Here's how the part is built. I have some questions about the finished solid (model axes, mm). A direction names the side the tool comes from. Round coordinates to 2 decimals unless told otherwise and drop trailing zeros. Order: outer loops, then holes, each group sorted by start corner. A loop starts at its lowest first (then second) coordinate and runs counter-clockwise, first axis right, second up.
```python
from build123d import *

# Parameters (mm, degrees)
SKETCH_1_W                = 24.86
SKETCH_1_H                = 41.68
SKETCH_1_R                = 0.75
EXTRUDE_2_DEPTH           = 2
SKETCH_4_W                = 2.869231424
SKETCH_4_H                = 4.001531821
SKETCH_4_W_2              = 2.43
SKETCH_4_H_2              = 4
EXTRUDE_3_DEPTH           = 24
SKETCH_8_W                = 3.310255182
SKETCH_8_H                = 4.675588029
SKETCH_8_W_2              = 3.47
EXTRUDE_5_DEPTH           = 16.03
FILLET_5_R                = 2.4
FILLET_6_R                = 2.4
FILLET_7_R                = 2.4
FILLET_8_R                = 2.4
CUT_EXTRUDE_7_DEPTH       = 16.03
CUT_EXTRUDE_7_DEPTH_BACK  = 16.03
SKETCH_13_R               = 1.236878532
CUT_EXTRUDE_8_DEPTH       = 16.03
CUT_EXTRUDE_8_DEPTH_BACK  = 16.03
SKETCH_5_R                = 1.45
CUT_EXTRUDE_9_DEPTH       = 16.03
CUT_EXTRUDE_9_DEPTH_BACK  = 16.03
SKETCH_14_R               = 1.4
SKETCH_16_W               = 16.135324728
SKETCH_16_H               = 3.096678483
EXTRUDE_8_DEPTH           = 10
FILLET_10_R               = 5
FILLET_13_R               = 5
SKETCH_17_W               = 2.433704545
SKETCH_17_H               = 5.946026496
SKETCH_17_W_2             = 1.564461462
SKETCH_17_H_2             = 6
EXTRUDE_9_DEPTH           = 15
CHAMFER_1_SIZE            = 10
CHAMFER_2_SIZE            = 10
CUT_EXTRUDE_16_DEPTH      = 10
CUT_EXTRUDE_16_DEPTH_BACK = 10
SKETCH_19_W               = 2.68
SKETCH_19_H               = 23.433804394
CUT_EXTRUDE_17_DEPTH      = 10
CUT_EXTRUDE_17_DEPTH_BACK = 10
SKETCH_18_W               = 2.24898196
SKETCH_18_H               = 30.410340658
FILLET_17_R               = 2
FILLET_18_R               = 2
FILLET_19_R               = 1


with BuildPart() as part:
    # 草图1 → 凸台-拉伸2 (new body)
    with BuildSketch(Plane(origin=(0, 0, 0), x_dir=(1, 0, 0), z_dir=(0, 1, 0))):
        Rectangle(SKETCH_1_W, SKETCH_1_H)
        with Locations(Location((-10.842762007, 19.642978565, 0), (0, 0, 270))):
            Circle(SKETCH_1_R, mode=Mode.SUBTRACT)
        with Locations(Location((10.87870886, 19.719816311, 0), (0, 0, 270))):
            Circle(SKETCH_1_R, mode=Mode.SUBTRACT)
        with Locations(Location((-10.713936696, -19.568538996, 0), (0, 0, 270))):
            Circle(SKETCH_1_R, mode=Mode.SUBTRACT)
        with Locations(Location((10.87870886, -19.568538996, 0), (0, 0, 270))):
            Circle(SKETCH_1_R, mode=Mode.SUBTRACT)
    extrude(amount=EXTRUDE_2_DEPTH)

    # 草图4 → 凸台-拉伸3 (add)
    with BuildSketch(Plane(origin=(0, 0, 0), x_dir=(1, 0, 0), z_dir=(0, 1, 0))):
        with Locations((-10.995384288, -16.41923409)):
            Rectangle(SKETCH_4_W, SKETCH_4_H)
        with Locations((11.215, -16.42)):
            Rectangle(SKETCH_4_W_2, SKETCH_4_H_2)
    extrude(amount=EXTRUDE_3_DEPTH)

    # 草图8 → 凸台-拉伸5 (add)
    with BuildSketch(Plane(origin=(0, 0, 0), x_dir=(1, 0, 0), z_dir=(0, 1, 0))):
        with Locations((-1.655127591, 18.102205985)):
            Rectangle(SKETCH_8_W, SKETCH_8_H)
        with Locations((4.770502505, 18.102205985)):
            Rectangle(SKETCH_8_W_2, SKETCH_8_H)
    extrude(amount=EXTRUDE_5_DEPTH)

    # 圆角5
    fillet_5_edges = [part.edges().sort_by_distance(p)[0] for p in [
        (-1.655127591, 16.03, -15.764411971),
    ]]
    fillet(fillet_5_edges, radius=FILLET_5_R)

    # 圆角6
    fillet_6_edges = [part.edges().sort_by_distance(p)[0] for p in [
        (4.770502505, 16.03, -15.764411971),
    ]]
    fillet(fillet_6_edges, radius=FILLET_6_R)

    # 圆角7
    # the kernel refuses this fillet: 2.4 mm, written as the material it takes off along each edge
    with BuildSketch(Plane(origin=(-2.956430437, 16.03, -20.44), x_dir=(0, 0, 1), z_dir=(1, 0, 0))) as fillet_7_piece_1_section:
        with BuildLine():
            CenterArc((2.4, 2.396773177), FILLET_7_R, 180, 87.028551133)
            Line((0, 2.396773177), (0, 0))
            Line((0, 0), (2.275588029, 0))
        make_face()
    fillet_7_piece_1 = extrude(amount=15.453865884, mode=Mode.PRIVATE)
    fillet_7_piece_1 = split(fillet_7_piece_1, bisect_by=Plane(origin=(0, 16.03, -20.44), z_dir=(1, 0, 0)), keep=Keep.TOP, mode=Mode.PRIVATE)
    add(fillet_7_piece_1, mode=Mode.SUBTRACT)

    # 圆角8
    # the kernel refuses this fillet: 2.4 mm, written as the material it takes off along each edge
    with BuildSketch(Plane(origin=(-9.302188124, 16.03, -20.44), x_dir=(0, 0, 1), z_dir=(1, 0, 0))) as fillet_8_piece_1:
        with BuildLine():
            CenterArc((2.4, 2.396773177), FILLET_8_R, 180, 87.028551133)
            Line((0, 2.396773177), (-0.048, 2.396773177))
            Line((-0.048, 2.396773177), (-0.048, 0))
            Line((-0.048, 0), (0, -0.048))
            ThreePointArc((0, -0.048), (1.137794014, -0.048), (2.273099789, -0.047935464))
            Line((2.273099789, -0.047935464), (2.275588029, 0))
        make_face()
    extrude(amount=15.294121066, mode=Mode.SUBTRACT)

    # 草图13 → 切除-拉伸7 (cut, two sides: drawn at the far end of the back side and taken through both)
    with BuildSketch(Plane(origin=(0, 0, 0), x_dir=(0, 0, -1), z_dir=(1, 0, 0)).offset(-CUT_EXTRUDE_7_DEPTH_BACK)):
        with Locations(Location((18.052862707, 13.197698645, 0), (0, 0, 180))):
            Circle(SKETCH_13_R)
    extrude(amount=CUT_EXTRUDE_7_DEPTH + CUT_EXTRUDE_7_DEPTH_BACK, mode=Mode.SUBTRACT)

    # 草图5 → 切除-拉伸8 (cut, two sides: drawn at the far end of the back side and taken through both)
    with BuildSketch(Plane(origin=(0, 0, 0), x_dir=(0, 0, -1), z_dir=(1, 0, 0)).offset(-CUT_EXTRUDE_8_DEPTH_BACK)):
        with Locations(Location((-16.419309005, 4.2, 0), (0, 0, 180))):
            Circle(SKETCH_5_R)
    extrude(amount=CUT_EXTRUDE_8_DEPTH + CUT_EXTRUDE_8_DEPTH_BACK, mode=Mode.SUBTRACT)

    # 草图14 → 切除-拉伸9 (cut, two sides: drawn at the far end of the back side and taken through both)
    with BuildSketch(Plane(origin=(0, 0, 0), x_dir=(0, 0, -1), z_dir=(1, 0, 0)).offset(-CUT_EXTRUDE_9_DEPTH_BACK)):
        with Locations(Location((-16.419309005, 22.241125132, 0), (0, 0, 180))):
            Circle(SKETCH_14_R)
    extrude(amount=CUT_EXTRUDE_9_DEPTH + CUT_EXTRUDE_9_DEPTH_BACK, mode=Mode.SUBTRACT)

    # 草图16 → 凸台-拉伸8 (add)
    with BuildSketch(Plane(origin=(0, 0, 0), x_dir=(1, 0, 0), z_dir=(0, 1, 0))):
        with Locations((1.276700778, 17.221878583)):
            Rectangle(SKETCH_16_W, SKETCH_16_H)
    extrude(amount=EXTRUDE_8_DEPTH)

    # 圆角10
    fillet_10_edges = [part.edges().sort_by_distance(p)[0] for p in [
        (-6.790961586, 10, -17.221878582),
    ]]
    fillet(fillet_10_edges, radius=FILLET_10_R)

    # 圆角13
    fillet_13_edges = [part.edges().sort_by_distance(p)[0] for p in [
        (9.344363142, 10, -17.221878582),
    ]]
    fillet(fillet_13_edges, radius=FILLET_13_R)

    # 草图17 → 凸台-拉伸9 (add)
    with BuildSketch(Plane(origin=(0, 0, 0), x_dir=(1, 0, 0), z_dir=(0, 1, 0))):
        with Locations((-11.213147728, -11.445454931)):
            Rectangle(SKETCH_17_W, SKETCH_17_H)
        with Locations((11.647769269, -11.42)):
            Rectangle(SKETCH_17_W_2, SKETCH_17_H_2)
    extrude(amount=EXTRUDE_9_DEPTH)

    # 倒角1
    # the kernel refuses this chamfer: 10 mm, written as the material it takes off along each edge
    with BuildSketch(Plane(origin=(-38.14682988, 15, 8.472441683), x_dir=(0, 0, 1), z_dir=(1, 0, 0))) as chamfer_1_piece_1_section:
        Polygon((CHAMFER_1_SIZE, 0), (0, CHAMFER_1_SIZE), (0, 0), align=None)
    chamfer_1_piece_1 = extrude(amount=53.867364305, mode=Mode.PRIVATE)
    chamfer_1_piece_1 = split(chamfer_1_piece_1, bisect_by=Plane(origin=(-38.14682988, 15, 14.418468179), z_dir=(0, 0, -1)), keep=Keep.TOP, mode=Mode.PRIVATE)
    chamfer_1_piece_1 = split(chamfer_1_piece_1, bisect_by=Plane(origin=(10, 15, 8.472441683), z_dir=(-1, 0, 0)), keep=Keep.TOP, mode=Mode.PRIVATE)
    add(chamfer_1_piece_1, mode=Mode.SUBTRACT)

    # 倒角2
    # the kernel refuses this chamfer: 10 mm, written as the material it takes off along each edge
    with BuildSketch(Plane(origin=(38.14682988, 15, 8.42), x_dir=(0, 0, 1), z_dir=(-1, 0, 0))) as chamfer_2_piece_1_section:
        Polygon((CHAMFER_2_SIZE, 0), (0, -CHAMFER_2_SIZE), (0, 0), align=None)
    chamfer_2_piece_1 = extrude(amount=52.998121222, mode=Mode.PRIVATE)
    chamfer_2_piece_1 = split(chamfer_2_piece_1, bisect_by=Plane(origin=(38.14682988, 15, 14.42), z_dir=(0, 0, -1)), keep=Keep.TOP, mode=Mode.PRIVATE)
    chamfer_2_piece_1 = split(chamfer_2_piece_1, bisect_by=Plane(origin=(10, 15, 8.42), z_dir=(1, 0, 0)), keep=Keep.TOP, mode=Mode.PRIVATE)
    add(chamfer_2_piece_1, mode=Mode.SUBTRACT)

    # 草图19 → 切除-拉伸16 (cut, two sides: drawn at the far end of the back side and taken through both)
    with BuildSketch(Plane(origin=(0, 0, 0), x_dir=(1, 0, 0), z_dir=(0, 1, 0)).offset(-CUT_EXTRUDE_16_DEPTH_BACK)):
        with Locations((-11.09, 6.483097803)):
            Rectangle(SKETCH_19_W, SKETCH_19_H)
    extrude(amount=CUT_EXTRUDE_16_DEPTH + CUT_EXTRUDE_16_DEPTH_BACK, mode=Mode.SUBTRACT)

    # 草图18 → 切除-拉伸17 (cut, two sides: drawn at the far end of the back side and taken through both)
    with BuildSketch(Plane(origin=(0, 0, 0), x_dir=(1, 0, 0), z_dir=(0, 1, 0)).offset(-CUT_EXTRUDE_17_DEPTH_BACK)):
        with Locations((11.30550902, 2.994829671)):
            Rectangle(SKETCH_18_W, SKETCH_18_H)
    extrude(amount=CUT_EXTRUDE_17_DEPTH + CUT_EXTRUDE_17_DEPTH_BACK, mode=Mode.SUBTRACT)

    # 圆角17
    fillet_17_edges = [part.edges().sort_by_distance(p)[0] for p in [
        (12.43, 1, -18.2),
    ]]
    fillet(fillet_17_edges, radius=FILLET_17_R)

    # 圆角18
    fillet_18_edges = [part.edges().sort_by_distance(p)[0] for p in [
        (-12.43, 1, -18.2),
    ]]
    fillet(fillet_18_edges, radius=FILLET_18_R)

    # 圆角19
    fillet_19_edges = [part.edges().sort_by_distance(p)[0] for p in [
        (10.18101804, 1, -18.2),
        (10.18101804, 1, 12.210340658),
        (-12.43, 1, 5.233804394),
        (-9.75, 1, 5.233804394),
    ]]
    fillet(fillet_19_edges, radius=FILLET_19_R)


solid = part.part
```
1. If we section it at B-B, the plane y = 4.2: State how many separate pieces and enclosed holes the cut face has, and give its area (3 significant figures).
Evaluation:
separate pieces: 5
enclosed holes: 0
area: 85.1 mm2
2. I'm going to push flat-ended pins straight in: P1, Ø1, axis at x = 4, y = 9.5, coming from the -Z side; P2, Ø2.5, axis at y = 3, z = -16.5, coming from the +X side; P3, Ø2.5, axis at x = 10.5, y = 8.5, coming from the -Z side; P4, Ø3, axis at x = -8, y = 20.5, coming from the -Z side. Where does each tip first touch, or does it pass through?
Evaluation:
P1: stops at z = -20.44
P2: stops at x = 10.18
P3: stops at z = 12.16
P4: passes through
3. I need wall thicknesses on probe 1 along X at (y, z) = (11.25, 17); probe 2 along X at (y, z) = (10.5, -17.5); probe 3 along Y at (x, z) = (-1, -15.5). Which ranges of each line are inside material? Lowest first, please.
Evaluation:
probe 1: x = -12.43 to -9.56, 10 to 12.43
probe 2: x = -3.31 to 0, 3.04 to 6.51
probe 3: y = 0 to 2
4. If we mould it in two halves opening along X, with no side actions, what happens to faces 4 (the flat face through (-12.43, 8, 14)), 5 (the flat face through (0, 0, 0)), 6 (the cylindrical face through (-11.17, 0.986, 18.973))? For each: released by +X, released by -X, zero draft, split by the parting line, or undercut.
Evaluation:
face 4: released by -X
face 5: zero draft
face 6: undercut
5. If we section it at D-D, the plane z = 13: Write out the boundary of the cut face in (x, y).
Evaluation:
outline: (-12.43, 0) - (12.43, 0) - (12.43, 9.58) - (10.87, 9.58) - (10.87, 2) - (-10, 2) - (-10, 9.53) - (-12.43, 9.53) - close
6. If we section it at A-A, the plane y = 19: Write out the boundary of the cut face in (x, z), and give its area (3 significant figures).
Evaluation:
outline: (-12.43, 14.42) - (-9.56, 14.42) - (-9.56, 18.42) - (-12.43, 18.42) - close; (10, 14.42) - (12.43, 14.42) - (12.43, 18.42) - (10, 18.42) - close
area: 21.2 mm2
7. If we section it at C-C, the plane x = 6: Write out the boundary of the cut face in (y, z), and give its area (3 significant figures).
Evaluation:
outline: (0, -20.84) - (2, -20.84) - (2, -20.44) - (13.63, -20.44) arc R2.4 ccw to (16.03, -18.16) arc R2.4 ccw to (13.63, -15.76) - (9.72, -15.76) - (9.72, -15.67) - (2, -15.67) - (2, 20.84) - (0, 20.84) - close; hole circle Ø2.47 at (13.2, -18.05)
area: 142 mm2
8. On a 3-axis mill with a long thin cutter (end or side, diameter ignored), from which of +Z, -Z, +X, -X, +Y, -Y can I reach the whole of each face in a straight line? I mean faces 1 (the flat face through (-3.31, 10, -19)), 2 (the flat face through (-9.75, 1, -7)), 3 (the flat face through (12, 4, 12.21)). Say none if no direction works.
Evaluation:
face 1: -Z, -X, +Y
face 2: -X, +Y, -Y
face 3: +X, +Y, -Y
